Geometry: final body of the model. Coordinates: model frame, mm. A direction names the side the tool comes from. Give positions to 0.01 mm unless a question says otherwise; leave off trailing zeros. Write each loop counter-clockwise with the first axis right and the second up, starting at its lowest first coordinate (ties: lowest second). Pieces come first, ordered by that corner, then holes.
from build123d import *

# Parameters (mm, degrees)
SKETCH2_W             = 80
SKETCH2_H             = 40
BOSS_EXTRUDE1_DEPTH   = 8
SKETCH3_R             = 2.5
BOSS_EXTRUDE2_DEPTH   = 9
SKETCH4_R             = 2.5
BOSS_EXTRUDE3_DEPTH   = 9
SKETCH5_R             = 2.5
BOSS_EXTRUDE4_DEPTH   = 9
CUT_EXTRUDE1_DEPTH    = 10
FILLET5_R             = 5
FILLET6_R             = 2.5
SKETCH8_W             = 8
SKETCH8_H             = 8
BOSS_EXTRUDE5_DEPTH   = 4
FILLET7_R             = 3.9
M3_CLEARANCE_HOLE1_D  = 3.4
M2X0_4_TAPPED_HOLE1_D = 1.6
FILLET7_OF_MIRROR1_R  = 3.9
SKETCH13_W            = 18.895911776
SKETCH13_H            = 64.667980446
CUT_EXTRUDE2_DEPTH    = 10


with BuildPart() as part:
    # Sketch2 → Boss-Extrude1 (new body)
    with BuildSketch(Plane(origin=(0, 0, 0), x_dir=(0, 0, -1), z_dir=(1, 0, 0))):
        with Locations((0, 20)):
            Rectangle(SKETCH2_W, SKETCH2_H)
    extrude(amount=BOSS_EXTRUDE1_DEPTH)

    # Sketch3 → Boss-Extrude2 (add)
    with BuildSketch(Plane(origin=(8, 0, 0), x_dir=(0, 0, -1), z_dir=(1, 0, 0))):
        with Locations((-36, 20)):
            Circle(SKETCH3_R)
        with Locations((-21, 20)):
            Circle(SKETCH3_R)
    extrude(amount=-BOSS_EXTRUDE2_DEPTH)

    # Sketch4 → Boss-Extrude3 (add)
    with BuildSketch(Plane(origin=(8, 0, 0), x_dir=(0, 0, -1), z_dir=(1, 0, 0))):
        with Locations((36, 20)):
            Circle(SKETCH4_R)
        with Locations((19, 32.6)):
            Circle(SKETCH4_R)
    extrude(amount=-BOSS_EXTRUDE3_DEPTH)

    # Sketch5 → Boss-Extrude4 (add)
    with BuildSketch(Plane(origin=(8, 0, 0), x_dir=(0, 0, -1), z_dir=(1, 0, 0))):
        with Locations((-10.5, 20)):
            Circle(SKETCH5_R)
        with Locations((10.5, 20)):
            Circle(SKETCH5_R)
        with Locations((10.5, 32.5)):
            Circle(SKETCH5_R)
        with Locations((-10.5, 32.5)):
            Circle(SKETCH5_R)
    extrude(amount=-BOSS_EXTRUDE4_DEPTH)

    # Sketch7 → Cut-Extrude1 (cut, through all)
    with BuildSketch(Plane(origin=(8, 0, 0), x_dir=(0, 0, -1), z_dir=(1, 0, 0))):
        Polygon((-31.8, 0), (-40, 16), (-47.08718472, 13.485117516), (-40, -21.908315756), (60.433184959, -20.412978779), (53.645426669, 13.485117516), (40, 16), (31.8, 0), (12.5, 0), (12.5, 17.5), (-12.5, 17.5), (-12.5, 0), align=None)
        Polygon((-40, 30), (-17, 30), (-17, 35.1), (40, 35.1), (58.962780813, 50.466125935), (-17, 44.25101618), (-17, 56.378048051), (-45.880127829, 54.443581987), align=None)
    extrude(amount=-CUT_EXTRUDE1_DEPTH, mode=Mode.SUBTRACT)

    # Fillet5
    fillet5_edges = [part.edges().sort_by_distance(p)[0] for p in [
        (4, 30, 40),
        (4, 35.1, -40),
        (4, 17.5, 12.5),
        (4, 17.5, -12.5),
        (4, 16, -40),
        (4, 16, 40),
    ]]
    fillet(fillet5_edges, radius=FILLET5_R)

    # Fillet6
    fillet6_edges = [part.edges().sort_by_distance(p)[0] for p in [
        (4, 35.1, 17),
        (4, 30, 17),
    ]]
    fillet(fillet6_edges, radius=FILLET6_R)

    # Sketch8 → Boss-Extrude5 (add)
    with BuildSketch(Plane(origin=(0, 0, 0), x_dir=(1, 0, 0), z_dir=(0, 1, 0))):
        with Locations((12, -24)):
            Rectangle(SKETCH8_W, SKETCH8_H)
        with Locations((12, 24)):
            Rectangle(SKETCH8_W, SKETCH8_H)
    boss_extrude5 = extrude(amount=BOSS_EXTRUDE5_DEPTH)

    # Fillet7
    fillet7_edges = [part.edges().sort_by_distance(p)[0] for p in [
        (16, 2, -20),
        (16, 2, -28),
        (16, 2, 28),
        (16, 2, 20),
    ]]
    fillet(fillet7_edges, radius=FILLET7_R)

    # M3 Clearance Hole1 (through all)
    with Locations(Plane(origin=(0, 4, 0), x_dir=(1, 0, 0), z_dir=(0, 1, 0))):
        with Locations((12, -24), (-4, -24), (-4, 24), (12, 24)):
            m3_clearance_hole1 = Hole(M3_CLEARANCE_HOLE1_D / 2)

    # M2x0.4 Tapped Hole1 (through all)
    with Locations(Plane.ZY.offset(1)):
        with Locations((-19, 32.6), (-36, 20), (-10.5, 32.5), (-10.5, 20), (10.5, 20), (10.5, 32.5), (21, 20), (36, 20)):
            Hole(M2X0_4_TAPPED_HOLE1_D / 2)

    # Mirror1: Boss-Extrude5, M3 Clearance Hole1 across plane
    add(boss_extrude5.mirror(Plane(origin=(4, 0, 0), x_dir=(0, 0, 1), z_dir=(1, 0, 0))))
    add(m3_clearance_hole1.mirror(Plane(origin=(4, 0, 0), x_dir=(0, 0, 1), z_dir=(1, 0, 0))), mode=Mode.SUBTRACT)

    # Fillet7 of Mirror1
    fillet7_of_mirror1_edges = [part.edges().sort_by_distance(p)[0] for p in [
        (-8, 2, -20),
        (-8, 2, -28),
        (-8, 2, 28),
        (-8, 2, 20),
    ]]
    fillet(fillet7_of_mirror1_edges, radius=FILLET7_OF_MIRROR1_R)

    # Sketch13 → Cut-Extrude2 (cut)
    with BuildSketch(Plane(origin=(0, 0, 0), x_dir=(1, 0, 0), z_dir=(0, 1, 0))):
        with Locations((17.447955888, 0.533990223)):
            Rectangle(SKETCH13_W, SKETCH13_H)
    extrude(amount=CUT_EXTRUDE2_DEPTH, mode=Mode.SUBTRACT)


solid = part.part
Q1. Pin query (flat end, axial travel): P1, Ø8, axis at x = 6, z = 14, coming from the -Y side; P2, Ø5.5, axis at y = 33.5, z = -9.5, coming from the -X side; P3, Ø6.5, axis at x = 5, z = 3, coming from the -Y side; P4, Ø4, axis at x = 4, z = 29, coming from the +Y side. Return the tip coordinate at first contact, or that it passes through.
Filled sheet:
P1: stops at y = 0
P2: stops at x = -1
P3: stops at y = 17.5
P4: stops at y = 30
Q2. Section B-B on y = 10.5. Output: boundary loops of the cut face in (x, z).
Filled sheet:
outline: (0, -37.18) - (8, -37.18) - (8, -12.5) - (0, -12.5) - close; (0, 12.5) - (8, 12.5) - (8, 37.18) - (0, 37.18) - close
Q3. Section D-D on z = 21. Output: boundary loops of the cut face in (x, y).
Filled sheet:
outline: (-6.71, 0) - (8, 0) - (8, 19.2) - (-1, 19.2) - (-1, 17.5) - (0, 17.5) - (0, 4) - (-6.71, 4) - close; (-1, 20.8) - (8, 20.8) - (8, 30) - (0, 30) - (0, 22.5) - (-1, 22.5) - close
Q4. Access query for faces 1 (the flat face through (-2, 2, 20)), 2 (the flat face through (-1, 21, 22)), 3 (the flat face through (0, 18, 1)). Directions: +Z, -Z, +X, -X, +Y, -Y. A direction counts if a zero-diameter tool reaches every point of the face in a straight line with its end or side. Return the directions, or none.
Filled sheet:
face 1: -X, -Y
face 2: +Z, -Z, -X, +Y
face 3: -X
Q5. Section A-A on x = 6.25. Count the separate pieces of the cut face and the enclosed holes in it, plus the area to 3 significant figures.
Filled sheet:
separate pieces: 1
enclosed holes: 8
area: 2,110 mm2
Q6. Ray query, line 1 along Z through (x, y) = (-4, 2.9); line 2 along X through (y, z) = (23, -1.5); line 3 along Y through (x, z) = (1.75, 21). Return the intervals inside material, ascending.
Filled sheet:
line 1: z = -28 to -25.7, -22.3 to -20, 20 to 22.3, 25.7 to 28
line 2: x = 0 to 8
line 3: y = 0 to 19.2, 20.8 to 30
Q7. Pull-direction query (Y, two-part tool) for faces 4 (the cylindrical face through (3.94, 33.6, -38.57)), 5 (the flat face through (4, 6, -12.5)), 6 (the cylindrical face through (3.563, 19.694, 35.261)); classes: released by +Y, released by -Y, zero draft, split by the parting line, or undercut.
Filled sheet:
face 4: released by +Y
face 5: zero draft
face 6: undercut
Q8. Section C-C on x = -6.5. Output: boundary loops of the cut face in (y, z).
Filled sheet:
outline: (0, -27.17) - (4, -27.17) - (4, -20.83) - (0, -20.83) - close; (0, 20.83) - (4, 20.83) - (4, 27.17) - (0, 27.17) - close
